Geometry check sheet. Reference: the model listing, model coordinates, mm. A direction names the side the tool comes from. Coordinates: 2 decimals unless noted, no trailing zeros. Write each loop counter-clockwise with the first axis right and the second up, starting at its lowest first coordinate (ties: lowest second). Pieces come first, ordered by that corner, then holes. Notation, with made-up numbers: (64, 86.5) -> (106, 86.5) arc R9 ccw to (106, 97.5) -> close; hole circle Ø11 at (1, 16.25). An arc over 180 degrees is marked (long way). Answer as CSV lines item,"result".
Autodesk Inventor part; units mm, degrees
ref_plane "YZ Plane" through (0, 0, 0) normal (1, 0, 0) x (0, 1, 0)
ref_plane "XZ Plane" through (0, 0, 0) normal (0, 1, 0) x (-1, 0, 0)
ref_plane "XY Plane" through (0, 0, 0) normal (0, 0, 1) x (1, 0, 0)
sketch "Sketch1" plane through (0, 0, 0) normal (0, 1, 0) x (-1, 0, 0)
  line L0 (0, 0) -> (-98, 0)
  line L1 (-98, 0) -> (-98, -53.377)
  line L2 (-98, -53.377) -> (0, -53.377)
  line L3 (0, -53.377) -> (0, 0)
  line L4 (-98, -53.377) -> (0, 0) construction
  dimension "d0" = 98
  dimension "d1" = 53.377
extrude "Extrusion1" add sketch "Sketch1" along normal blind 6
sketch "Sketch2" plane through (0, 6, 0) normal (0, 1, 0) x (1, 0, 0)
  line L0 (98, 0) -> (98, 53.377)
  line L1 (0, 0) -> (98, 0)
  line L2 (98, 53.377) -> (92, 53.377)
  line L3 (92, 53.377) -> (92, 0)
  line L4 (92, 0) -> (98, 0)
  line L5 (98, 0) -> (98, 53.377)
  line L6 (0, 53.377) -> (6, 53.377)
  line L7 (6, 53.377) -> (6, 0)
  line L8 (6, 0) -> (0, 0)
  line L9 (0, 0) -> (0, 53.377)
  dimension "d4" = 6
  dimension "d5" = 6
extrude "Extrusion2" add sketch "Sketch2" along normal blind 40
sketch "Sketch3" plane through (0, 0, -53.377) normal (-1, 0, 0) x (0, 0, 1)
  arc A0 (41.0993, 20) -> (12.1996, 20) centre (26.6494, 20.0723) ccw construction
  arc A1 (43.3493, 19.9888) -> (9.9496, 19.9888) centre (26.6494, 20.0723) ccw
  arc A2 (38.8493, 20.0113) -> (14.4496, 20.0113) centre (26.6494, 20.0723) ccw
  arc A3 (38.8493, 20.0113) -> (43.3493, 19.9888) centre (41.0993, 20) ccw
  arc A4 (9.9496, 19.9888) -> (14.4496, 20.0113) centre (12.1996, 20) ccw
  circle A5 centre (26.6495, 20) radius 2.25
  circle A6 centre (41.0993, 20) radius 2.25
  circle A7 centre (12.1996, 20) radius 2.25
  circle A8 centre (26.6494, 34.5224) radius 2.25
  point P0 (53.377, 0)
  dimension "d8" = 4.5
  dimension "d9" = 4.5
  dimension "d36" = 14.45
extrude "Extrusion3" cut sketch "Sketch3" against normal blind 110 and the other way blind 12.5 contours A3 A6 A1 | A8 | A7 A4 | A5
sketch "Sketch4" plane through (0, 0, 0) normal (0, -1, 0) x (1, 0, 0)
  line L0 (98, -53.377) -> (92, -53.377) construction
  line L1 (98, -53.377) -> (0, 0) construction
  line L2 (64, -41.6885) -> (34, -41.6885)
  line L3 (34, -41.6885) -> (34, -11.6885)
  line L4 (34, -11.6885) -> (64, -11.6885)
  line L5 (64, -11.6885) -> (64, -41.6885)
  line L6 (64, -41.6885) -> (34, -11.6885) construction
  line L7 (34, -41.6885) -> (64, -11.6885) construction
  circle A0 centre (49, -26.6885) radius 11.75
  dimension "d16" = 30
  dimension "d17" = 30
  dimension "d18" = 23.5
extrude "Extrusion4" add sketch "Sketch4" along normal blind 30
sketch "Sketch5" plane through (34, 0, -11.6885) normal (0, 0, 1) x (1, 0, 0)
  line L0 (0, -30) -> (30, -30) construction
  line L1 (30, 0) -> (0, 0) construction
  circle A0 centre (15, -18) radius 1.75
  point P0 (-34, 0)
  dimension "d21" = 3.5
  dimension "d26" = 12
extrude "Extrusion5" cut sketch "Sketch5" against normal blind 33
sketch "Sketch7" plane through (34, 0, -41.6885) normal (-1, 0, 0) x (0, 0, 1)
  line L0 (0, 0) -> (0, -30) construction
  line L1 (30, 0) -> (30, -30) construction
  circle A0 centre (15, -18) radius 1.75
  line L2 (30, -30) -> (0, -30)
  point P0 (41.6885, 0)
  dimension "d31" = 3.5
  dimension "d32" = 12
extrude "Extrusion7" cut sketch "Sketch7" against normal blind 33
fillet "Fillet3" radius 6 16 edges at (0, 0, -26.6885) (98, 0, -26.6885) (64, -15, -41.6885) (34, -15, -41.6885) (49, 0, -41.6885) (34, 0, -26.6885) (34, -15, -11.6885) (49, 0, -11.6885) (64, -15, -11.6885) (64, 0, -26.6885) (6, 6, -26.6885) (92, 6, -26.6885) (95, 46, 0) (3, 46, 0) (3, 46, -53.377) (95, 46, -53.377)
properties part number "Drone_holder_base"
Item 1: Cross-section at C-C, the plane y = 29.5. Record the cut outline in (x, z), plus the area to 3 significant figures.
Responses:
outline,"(0, -53.38) -> (6, -53.38) -> (6, 0) -> (0, 0) -> close; (92, -53.38) -> (98, -53.38) -> (98, 0) -> (92, 0) -> close"
area,"641 mm2"
Item 2: Cross-section at A-A, the plane x = 49. Record the cut outline in (y, z), plus the area to 3 significant figures.
Responses:
outline,"(-30, -41.69) -> (-19.75, -41.69) -> (-19.75, -38.44) -> (-30, -38.44) -> close; (-30, -14.94) -> (-19.75, -14.94) -> (-19.75, -11.69) -> (-30, -11.69) -> close; (-16.25, -41.69) -> (-6, -41.69) arc R6 cw to (0, -47.69) -> (0, -53.38) -> (6, -53.38) -> (6, 0) -> (0, 0) -> (0, -5.69) arc R6 cw to (-6, -11.69) -> (-16.25, -11.69) -> (-16.25, -14.94) -> (0, -14.94) -> (0, -38.44) -> (-16.25, -38.44) -> close"
area,"508 mm2"
Item 3: Cross-section at B-B, the plane y = -18. Record the cut outline in (x, z).
Responses:
outline,"(34, -35.69) arc R6 ccw to (40, -41.69) -> (47.25, -41.69) -> (47.25, -38.31) arc R11.75 cw to (37.38, -28.44) -> (34, -28.44) -> close; (34, -24.94) -> (37.38, -24.94) arc R11.75 cw to (47.25, -15.07) -> (47.25, -11.69) -> (40, -11.69) arc R6 ccw to (34, -17.69) -> close; (50.75, -41.69) -> (58, -41.69) arc R6 ccw to (64, -35.69) -> (64, -28.44) -> (60.62, -28.44) arc R11.75 cw to (50.75, -38.31) -> close; (50.75, -15.07) arc R11.75 cw to (60.62, -24.94) -> (64, -24.94) -> (64, -17.69) arc R6 ccw to (58, -11.69) -> (50.75, -11.69) -> close"
Item 4: Set-up check for faces 4 (the cylindrical face through (2.96, 17.75, -41.22)), 5 (the flat face through (6, 29, -27)), 6 (the flat face through (50, 0, -50)), 7 (the flat face through (51, -18, -41.688)), 8 (the cylindrical face through (94.96, 44.29, -51.57)): record each of +Z, -Z, +X, -X, +Y, -Y from which the full face is reachable in a straight line by a thin tool's end or side.
Responses:
face 4,"+X, -X"
face 5,"+Z, -Z, +Y"
face 6,"-Y"
face 7,"-Z, +X, -X, -Y"
face 8,"-Z, +X, -X, +Y"
Item 5: Release check for a two-part mould opening along X. For faces 1 (the cylindrical face through (96.289, 1.804, -27.062)), 2 (the flat face through (50, 6, -26)), 3 (the cylindrical face through (2.96, 17.75, -12.34)) record: +X half, -X half, draft (parallel to the pull), parting line (faces both ways), or undercut.
Responses:
face 1,"+X half"
face 2,"undercut"
face 3,"draft"
Item 6: Depth check by flat-ended pin: pin 1 Ø14.5 at (x, y) = (49, -23) entering from -Z; pin 2 Ø6 at (y, z) = (20, -26.73) entering from +X; pin 3 Ø7 at (x, z) = (45.5, -31.5) entering from -Y; pin 4 Ø1.5 at (x, z) = (18.5, -16.5) entering from +Y. Enter the tip coordinate at first touch or a pass-through.
Responses:
pin 1,"stops at z = -41.69"
pin 2,"stops at x = 98"
pin 3,"stops at y = 0"
pin 4,"stops at y = 6"
Item 7: Thickness scan on probe 1 along Y at (x, z) = (49, -14.1); probe 2 along X at (y, z) = (34, -19.5); probe 3 along X at (y, z) = (-7, -16.5). Record the ranges inside material, lowest first.
Responses:
probe 1,"y = -30 to -19.75, -16.25 to 6"
probe 2,"x = 0 to 6, 92 to 98"
probe 3,"x = 34.12 to 43.15, 54.85 to 63.88"
Item 8: Cross-section at D-D, the plane y = -9.5. Record the cut outline in (x, z).
Responses:
outline,"(34, -35.69) arc R6 ccw to (40, -41.69) -> (58, -41.69) arc R6 ccw to (64, -35.69) -> (64, -17.69) arc R6 ccw to (58, -11.69) -> (40, -11.69) arc R6 ccw to (34, -17.69) -> close; hole circle Ø23.5 at (49, -26.69)"
